Print and shaded views of the part. All mm, measured from the part's lowest x, y and z. Round coordinates to 2 decimals unless told otherwise and drop trailing zeros. Loops run counter-clockwise (first coordinate to the right, second up) from the corner with the lowest first, then second, coordinate; pieces in that order, holes last. Notation, with made-up numbers: (-11, 8) -> (3, 8) arc R27 cw to (3, 37) -> close; hole circle Ø4 at (-1.75, 69). An arc over 180 degrees is marked (long way). Answer as CSV lines item,"result".
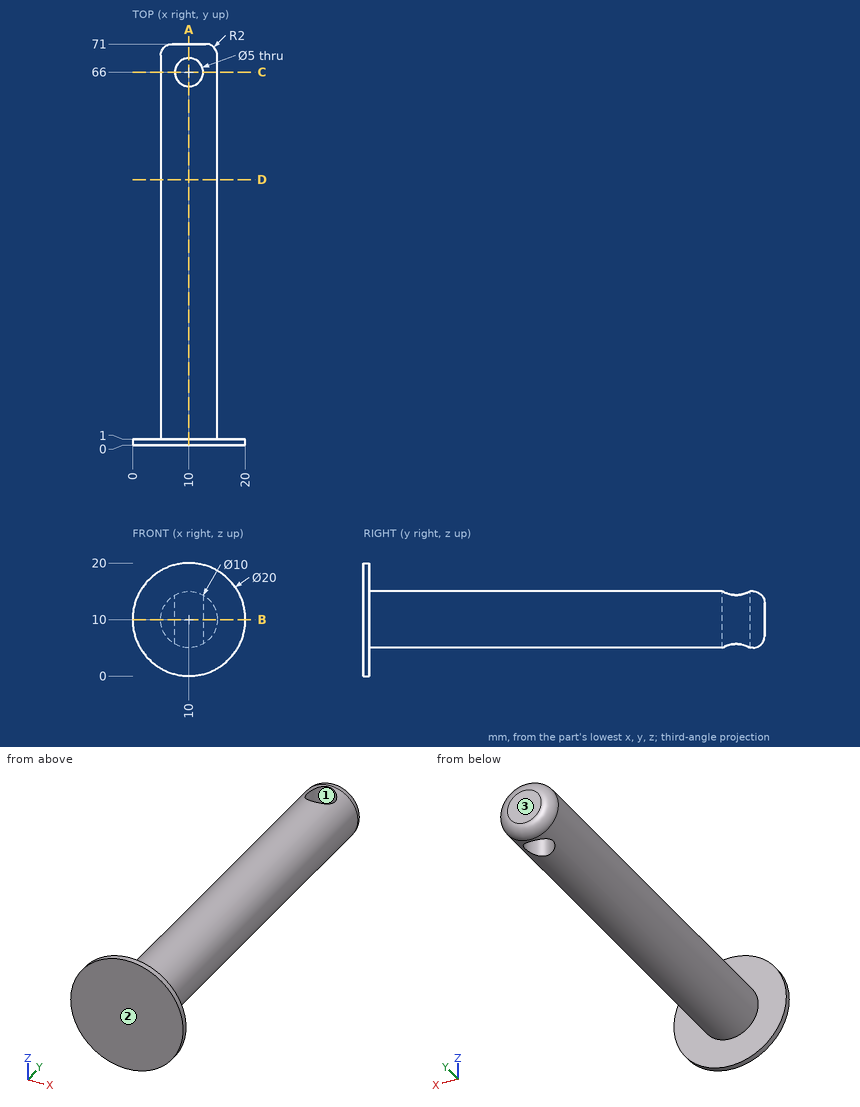
Q1. Saw through at C-C, the plane y = 66. Write the cut outline in (x, z).
Geometry results:
outline,"(7.5, 5.67) -> (7.5, 14.33) arc R5 ccw to start; (12.5, 5.67) arc R5 ccw to (12.5, 14.33) -> close"
Q2. Saw through at D-D, the plane y = 47. Write the cut outline in (x, z).
Geometry results:
outline,"circle Ø10 at (10, 10)"
Q3. Drill centre lines: line 1 along Y through (x, z) = (10, 8.75); line 2 along Z through (x, y) = (10.25, 5.5); line 3 along Y through (x, z) = (17.25, 9). Where is each one in solid material? Low to high.
Geometry results:
line 1,"0 to 63.5, 68.5 to 71"
line 2,"5.01 to 14.99"
line 3,"0 to 1"
Q4. Saw through at B-B, the plane z = 10. Write the cut outline in (x, y).
Geometry results:
outline,"(0, 0) -> (20, 0) -> (20, 1) -> (15, 1) -> (15, 69) arc R2 ccw to (13, 71) -> (7, 71) arc R2 ccw to (5, 69) -> (5, 1) -> (0, 1) -> close; hole circle Ø5 at (10, 66)"
Q5. Saw through at A-A, the plane x = 10. Write the cut outline in (y, z), then the cut area to 3 significant figures.
Geometry results:
outline,"(0, 0) -> (1, 0) -> (1, 5) -> (63.5, 5) -> (63.5, 15) -> (1, 15) -> (1, 20) -> (0, 20) -> close; (68.5, 5) -> (69, 5) arc R2 ccw to (71, 7) -> (71, 13) arc R2 ccw to (69, 15) -> (68.5, 15) -> close"
area,"668 mm2"
Q6. Drop flat-ended pins along their axis: P1, Ø2, axis at y = 8, z = 5.5, coming from the -X side; P2, Ø12, axis at x = 2.5, y = 53, coming from the -Z side; P3, Ø4, axis at y = 52, z = 15, coming from the -X side; P4, Ø4, axis at x = 10, y = 66, coming from the -Z side. Give the stop position or say it passes through.
Geometry results:
P1,"x = 6.43"
P2,"z = 5.23"
P3,"x = 6"
P4,"through"
Q7. Two-plate mould, pull along Y, no slides. Class the marked faces 1, 2 and 3: pulls with the +Y half, pulls with the -Y half, needs draft (parallel to the pull), parting line crosses it, or undercut.
Geometry results:
face 1,"undercut"
face 2,"pulls with the -Y half"
face 3,"pulls with the +Y half"
